Here's how the part is built. I have some questions about the finished solid (model axes, mm). A direction names the side the tool comes from. Round coordinates to 2 decimals unless told otherwise and drop trailing zeros. Order: outer loops, then holes, each group sorted by start corner. A loop starts at its lowest first (then second) coordinate and runs counter-clockwise, first axis right, second up. Notation, with made-up numbers: (-3.75, -6) -> (12.25, -6) arc R20 ccw to (12.25, 21) -> close; hole circle Ø1 at (88, -36). An arc over 180 degrees is marked (long way). Answer in a Markdown table with one row per item.
```python
from build123d import *

# Parameters (mm, degrees)
SKETCH1_W           = 130
SKETCH1_H           = 60
BOSS_EXTRUDE1_DEPTH = 2.5
SKETCH2_R           = 2.5
BOSS_EXTRUDE2_DEPTH = 4
SKETCH3_W           = 4
SKETCH3_H           = 37
BOSS_EXTRUDE3_DEPTH = 20
SKETCH4_W           = 4
SKETCH4_H           = 28
BOSS_EXTRUDE4_DEPTH = 18
SKETCH5_R           = 0.9
CUT_EXTRUDE1_DEPTH  = 145.069427708
SKETCH6_W           = 3
SKETCH6_H           = 3
SKETCH6_W_2         = 1.5
SKETCH6_W_3         = 2
CUT_EXTRUDE2_DEPTH  = 145.568322948
SKETCH7_W           = 20
SKETCH7_H           = 25
SKETCH7_W_2         = 8.5
SKETCH7_H_2         = 13.2
BOSS_EXTRUDE5_DEPTH = 6
SKETCH8_W           = 35
SKETCH8_H           = 4
BOSS_EXTRUDE6_DEPTH = 21
SKETCH9_W           = 3
SKETCH9_H           = 3
SKETCH9_W_2         = 2.5
CUT_EXTRUDE3_DEPTH  = 145.710054937
SKETCH11_W          = 77
SKETCH11_H          = 20.5
BOSS_EXTRUDE8_DEPTH = 3.75
SKETCH12_R          = 1.325
CUT_EXTRUDE4_DEPTH  = 146.09393509


with BuildPart() as part:
    # Sketch1 → Boss-Extrude1 (new body)
    with BuildSketch(Plane.XY):
        with Locations((65, 30)):
            Rectangle(SKETCH1_W, SKETCH1_H)
    extrude(amount=BOSS_EXTRUDE1_DEPTH)

    # Sketch2 → Boss-Extrude2 (add)
    with BuildSketch(Plane.XY.offset(2.5)):
        with Locations(Location((50, 7, 0), (0, 0, 180))):
            Circle(SKETCH2_R)
        with Locations(Location((105, 7, 0), (0, 0, 180))):
            Circle(SKETCH2_R)
        with Locations(Location((50, 53, 0), (0, 0, 180))):
            Circle(SKETCH2_R)
    extrude(amount=BOSS_EXTRUDE2_DEPTH)

    # Sketch3 → Boss-Extrude3 (add)
    with BuildSketch(Plane.XY.offset(2.5)):
        with Locations((112, 23.5)):
            Rectangle(SKETCH3_W, SKETCH3_H)
    extrude(amount=BOSS_EXTRUDE3_DEPTH)

    # Sketch4 → Boss-Extrude4 (add)
    with BuildSketch(Plane.XY.offset(2.5)):
        with Locations((123, 14)):
            Rectangle(SKETCH4_W, SKETCH4_H)
    extrude(amount=BOSS_EXTRUDE4_DEPTH)

    # Sketch5 → Cut-Extrude1 (cut, through all)
    with BuildSketch(Plane.XY.offset(6.5)):
        with Locations((105, 7)):
            Circle(SKETCH5_R)
        with Locations((50, 7)):
            Circle(SKETCH5_R)
        with Locations((50, 53)):
            Circle(SKETCH5_R)
    extrude(amount=-CUT_EXTRUDE1_DEPTH, mode=Mode.SUBTRACT)

    # Sketch6 → Cut-Extrude2 (cut, through all)
    with BuildSketch(Plane.XY.offset(2.5)):
        with Locations((108.5, 36.5)):
            Rectangle(SKETCH6_W, SKETCH6_H)
        with Locations((108.5, 9.5)):
            Rectangle(SKETCH6_W, SKETCH6_H)
        with Locations((120.25, 20.5)):
            Rectangle(SKETCH6_W_2, SKETCH6_H)
        with Locations((128, 20.5)):
            Rectangle(SKETCH6_W_3, SKETCH6_H)
        with Locations((128, 9.5)):
            Rectangle(SKETCH6_W_3, SKETCH6_H)
        with Locations((120.25, 9.5)):
            Rectangle(SKETCH6_W_2, SKETCH6_H)
        with Locations((117, 9.5)):
            Rectangle(SKETCH6_W_3, SKETCH6_H)
        with Locations((117.5, 36.5)):
            Rectangle(SKETCH6_W, SKETCH6_H)
    extrude(amount=-CUT_EXTRUDE2_DEPTH, mode=Mode.SUBTRACT)

    # Sketch7 → Boss-Extrude5 (add)
    with BuildSketch(Plane(origin=(130, 0, 0), x_dir=(0, 0, -1), z_dir=(1, 0, 0))):
        with Locations((-10, 47.5)):
            Rectangle(SKETCH7_W, SKETCH7_H)
        with Locations((-10, 49.4)):
            Rectangle(SKETCH7_W_2, SKETCH7_H_2, mode=Mode.SUBTRACT)
    extrude(amount=-BOSS_EXTRUDE5_DEPTH)

    # Sketch8 → Boss-Extrude6 (add)
    with BuildSketch(Plane.XY.offset(2.5)):
        with Locations((17.5, 49)):
            Rectangle(SKETCH8_W, SKETCH8_H)
        with Locations((17.5, 30)):
            Rectangle(SKETCH8_W, SKETCH8_H)
        with Locations((17.5, 11)):
            Rectangle(SKETCH8_W, SKETCH8_H)
    extrude(amount=BOSS_EXTRUDE6_DEPTH)

    # Sketch9 → Cut-Extrude3 (cut, through all)
    with BuildSketch(Plane.XY.offset(2.5)):
        with Locations((9.5, 14.5)):
            Rectangle(SKETCH9_W, SKETCH9_H)
        with Locations((25.5, 14.5)):
            Rectangle(SKETCH9_W, SKETCH9_H)
        with Locations((9.5, 33.5)):
            Rectangle(SKETCH9_W, SKETCH9_H)
        with Locations((25.5, 33.5)):
            Rectangle(SKETCH9_W, SKETCH9_H)
        with Locations((9.5, 52.5)):
            Rectangle(SKETCH9_W, SKETCH9_H)
        with Locations((25.5, 52.5)):
            Rectangle(SKETCH9_W, SKETCH9_H)
        with Locations((9.25, 5.5)):
            Rectangle(SKETCH9_W_2, SKETCH9_H)
        with Locations((9.25, 24.5)):
            Rectangle(SKETCH9_W_2, SKETCH9_H)
        with Locations((25.5, 24.5)):
            Rectangle(SKETCH9_W, SKETCH9_H)
        with Locations((25.5, 5.5)):
            Rectangle(SKETCH9_W, SKETCH9_H)
        with Locations((25.5, 43.5)):
            Rectangle(SKETCH9_W, SKETCH9_H)
        with Locations((9.25, 43.5)):
            Rectangle(SKETCH9_W_2, SKETCH9_H)
    extrude(amount=-CUT_EXTRUDE3_DEPTH, mode=Mode.SUBTRACT)

    # Sketch11 → Boss-Extrude8 (add)
    with BuildSketch(Plane.XZ):
        with Locations((86.5, 10.25)):
            Rectangle(SKETCH11_W, SKETCH11_H)
    extrude(amount=-BOSS_EXTRUDE8_DEPTH)

    # Sketch12 → Cut-Extrude4 (cut, through all)
    with BuildSketch(Plane.XZ):
        with Locations(Location((87.03, 13.12, 0), (0, 0, 270))):
            Circle(SKETCH12_R)
    extrude(amount=-CUT_EXTRUDE4_DEPTH, mode=Mode.SUBTRACT)


solid = part.part
```
1. Please list where these lines run through material, in increasing order: line 1 along Y through (x, z) = (21.5, 11); line 2 along Y through (x, z) = (50, 3.75); line 3 along X through (y, z) = (53, 4.5).
Numbers:
| item | result |
|---|---|
| line 1 | y = 9 to 13, 28 to 32, 47 to 51 |
| line 2 | y = 0 to 3.75, 4.5 to 6.1, 7.9 to 9.5, 50.5 to 52.1, 53.9 to 55.5 |
| line 3 | x = 47.5 to 49.1, 50.9 to 52.5, 124 to 130 |
2. For pin 1 Ø4 at (x, z) = (24.5, 6) entering from +Y; pin 2 Ø8 at (x, z) = (27.5, 7.5) entering from -Y; pin 3 Ø5 at (y, z) = (24.5, 6.5) entering from +X, each with a flat end and sliding along its axis, tell me the tip position at first contact or that it passes through.
Numbers:
| item | result |
|---|---|
| pin 1 | stops at y = 51 |
| pin 2 | stops at y = 9 |
| pin 3 | stops at x = 125 |
3. Suppose I cut it at A-A on z = 9. State how many separate pieces and enclosed holes the cut face has, then the cut area to 3 significant figures.
Numbers:
| item | result |
|---|---|
| separate pieces | 7 |
| enclosed holes | 0 |
| area | 1,020 mm2 |
4. Suppose I cut it at B-B on x = 87.03. Write out the boundary of the cut face in (y, z) (3 decimals), then the cut area to 3 significant figures.
Numbers:
| item | result |
|---|---|
| outline | (0, 0) -> (60, 0) -> (60, 2.5) -> (3.75, 2.5) -> (3.75, 11.795) -> (0, 11.795) -> close; (0, 14.445) -> (3.75, 14.445) -> (3.75, 20.5) -> (0, 20.5) -> close |
| area | 208 mm2 |
5. For faces 4 (the face through (64, 30, 0)), 5 (the face through (114, 23, 12)), 6 (the face through (25, 7, 1)), which set-ups out of +Z, -Z, +X, -X, +Y, -Y let a thin tool reach every point of the face, with its end or its side?
Numbers:
| item | result |
|---|---|
| face 4 | -Z, +X, -X, +Y, -Y |
| face 5 | +Z, +Y |
| face 6 | +Z, -Z |
6. Suppose I cut it at C-C on x = 36.5. Write out the boundary of the cut face in (y, z), then the cut area to 3 significant figures.
Numbers:
| item | result |
|---|---|
| outline | (0, 0) -> (60, 0) -> (60, 2.5) -> (0, 2.5) -> close |
| area | 150 mm2 |
7. We'd pull the mould along X, two halves only. Please class faces 1 (the face through (48.9, 53, 6.5)), 2 (the face through (10.5, 43, 1)), 3 (the face through (10.5, 24, 1)): released by +X, released by -X, zero draft, split by the parting line, or undercut.
Numbers:
| item | result |
|---|---|
| face 1 | zero draft |
| face 2 | undercut |
| face 3 | undercut |
